from build123d import *

# Parameters (mm, degrees)
SKETCH2_R               = 5
BOSS_EXTRUDE1_DEPTH     = 5
SKETCH3_R               = 12.5
BOSS_EXTRUDE2_DEPTH     = 1.5
CUT_EXTRUDE1_DEPTH      = 22.943108257
CUT_EXTRUDE1_DEPTH_BACK = 22.943108257
SKETCH5_R               = 4.4
BOSS_EXTRUDE3_DEPTH     = 4
CUT_EXTRUDE2_DEPTH      = 25.525496937
SKETCH7_R               = 1.25
CUT_EXTRUDE3_DEPTH      = 23.210438987
SKETCH9_R               = 2
CUT_EXTRUDE4_DEPTH      = 22.089096709


with BuildPart() as part:
    # Sketch2 → Boss-Extrude1 (new, symmetric)
    with BuildSketch(Plane(origin=(0, 0, 0), x_dir=(1, 0, 0), z_dir=(0, 1, 0))):
        with Locations(Location((0, 0, 0), (0, 0, 270))):
            Circle(SKETCH2_R)
    extrude(amount=BOSS_EXTRUDE1_DEPTH, both=True)

    # Sketch3 → Boss-Extrude2 (add)
    with BuildSketch(Plane(origin=(0, 5, 0), x_dir=(1, 0, 0), z_dir=(0, 1, 0))):
        with Locations(Location((0, 0, 0), (0, 0, 270))):
            Circle(SKETCH3_R)
    boss_extrude2 = extrude(amount=BOSS_EXTRUDE2_DEPTH)

    # Mirror1: Boss-Extrude2 across plane
    add(boss_extrude2.mirror(Plane.ZX))

    # Sketch4 → Cut-Extrude1 (cut, two sides: drawn at the far end of the back side and taken through both)
    with BuildSketch(Plane(origin=(0, 6.5, 0), x_dir=(1, 0, 0), z_dir=(0, 1, 0)).offset(-CUT_EXTRUDE1_DEPTH_BACK)):
        with BuildLine():
            Line((-1.92, 2.56), (1.92, 2.56))
            ThreePointArc((1.92, 2.56), (0, -3.2), (-1.92, 2.56))
        make_face()
    extrude(amount=CUT_EXTRUDE1_DEPTH + CUT_EXTRUDE1_DEPTH_BACK, mode=Mode.SUBTRACT)

    # Sketch5 → Boss-Extrude3 (add)
    with BuildSketch(Plane(origin=(0, 6.5, 0), x_dir=(1, 0, 0), z_dir=(0, 1, 0))):
        with Locations(Location((0, 0, 0), (0, 0, 270))):
            Circle(SKETCH5_R)
    extrude(amount=BOSS_EXTRUDE3_DEPTH)

    # Sketch6 → Cut-Extrude2 (cut, through all)
    with BuildSketch(Plane(origin=(0, 10.5, 0), x_dir=(1, 0, 0), z_dir=(0, 1, 0))):
        with BuildLine():
            Line((-1.92, 2.56), (1.92, 2.56))
            ThreePointArc((1.92, 2.56), (0, -3.2), (-1.92, 2.56))
        make_face()
    extrude(amount=-CUT_EXTRUDE2_DEPTH, mode=Mode.SUBTRACT)

    # Sketch7 → Cut-Extrude3 (cut, through all)
    with BuildSketch(Plane.XY.offset(-2.56)):
        with Locations((0, 8.3)):
            Circle(SKETCH7_R)
    extrude(amount=-CUT_EXTRUDE3_DEPTH, mode=Mode.SUBTRACT)

    # Sketch9 → Cut-Extrude4 (cut, through all)
    with BuildSketch(Plane.XZ.offset(-5)):
        with Locations(Location((0, 8, 0), (0, 0, 270))):
            Circle(SKETCH9_R)
    extrude(amount=-CUT_EXTRUDE4_DEPTH, mode=Mode.SUBTRACT)


solid = part.part
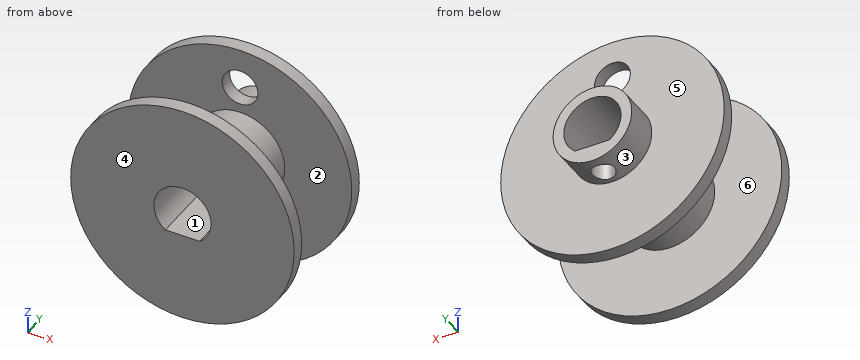
Input: part model. Units: mm. Frame: model coordinates. Face numbers are marked on the shaded views. A direction names the side the tool comes from. Round coordinates to 2 decimals unless told otherwise and drop trailing zeros. Order: outer loops, then holes, each group sorted by start corner. A loop starts at its lowest first (then second) coordinate and runs counter-clockwise, first axis right, second up. Notation, with made-up numbers: (60, 4.5) - (75, 4.5) arc R22 cw to (75, 35.5) - close; hole circle Ø9 at (80, 45). An arc over 180 degrees is marked (long way). Answer as a JSON object with one key per item and string values. Group by question number.
(1) Material intervals for probe 1 along Y at (x, z) = (2, -10.5); probe 2 along Y at (x, z) = (0, -3.85); probe 3 along Z at (x, y) = (-1.75, 6), sorted ascending. Write a range as from..to.
(2) Cut plane D-D (z = 8). Return loops of the section in (x, y), then the cut area to 3 significant figures.
(3) Cut plane B-B (z = 0). Return loops of the section in (x, y), then the cut area to 3 significant figures.
(4) Cut plane A-A (x = 7.5). Return loops of the section in (y, z).
(5) Draft query along X for the marked faces 1, 2 and 3. Return one class per face: released by +X, released by -X, zero draft, split by the parting line, or undercut.
(6) Reachability of the marked faces 4, 5 and 6 from +Z, -Z, +X, -X, +Y, -Y: full face, straight path, thin tool, end or side. Return the list, or none.
(7) Pin query (flat end, axial travel): P1, Ø3, axis at x = 0, y = 8.3, coming from the +Z side; P2, Ø1.5, axis at y = -0.5, z = -3.5, coming from the -X side; P3, Ø6.5, axis at x = 0, z = 8, coming from the +Y side; P4, Ø1.5, axis at x = -7.5, y = 3, coming from the +Z side. Return the tip coordinate at first contact, or that it passes through.
(8) Cut plane C-C (x = 0). Return loops of the section in (y, z).
Here are the results:
{
 "1": {"probe 1": "y = -6.5..-5, 5..6.5", "probe 2": "y = -6.5..7.05, 9.55..10.5", "probe 3": "z = -12.38..-2.56, 2.68..7.03, 8.97..12.38"},
 "2": {"outline": "(-9.6, -6.5) - (9.6, -6.5) - (9.6, -5) - (-9.6, -5) - close; (-9.6, 5) - (-2, 5) - (-2, 6.5) - (-9.6, 6.5) - close; (2, 5) - (9.6, 5) - (9.6, 6.5) - (2, 6.5) - close", "area": "51.6 mm^2"},
 "3": {"outline": "(-12.5, -6.5) - (-3.2, -6.5) - (-3.2, 10.5) - (-4.4, 10.5) - (-4.4, 6.5) - (-12.5, 6.5) - (-12.5, 5) - (-5, 5) - (-5, -5) - (-12.5, -5) - close; (3.2, -6.5) - (12.5, -6.5) - (12.5, -5) - (5, -5) - (5, 5) - (12.5, 5) - (12.5, 6.5) - (4.4, 6.5) - (4.4, 10.5) - (3.2, 10.5) - close", "area": "101 mm^2"},
 "4": {"outline": "(-6.5, -10) - (-5, -10) - (-5, 10) - (-6.5, 10) - close; (5, -10) - (6.5, -10) - (6.5, 10) - (5, 10) - close"},
 "5": {"face 1": "undercut", "face 2": "zero draft", "face 3": "split by the parting line"},
 "6": {"face 4": "+Z, -Z, +X, -X, -Y", "face 5": "+Y", "face 6": "none"},
 "7": {"P1": "stops at z = 4.4", "P2": "stops at x = -4.18", "P3": "stops at y = 6.5", "P4": "passes through"},
 "8": {"outline": "(-6.5, -12.5) - (-5, -12.5) - (-5, -5) - (5, -5) - (5, -12.5) - (6.5, -12.5) - (6.5, -4.4) - (7.05, -4.4) - (7.05, -2.56) - (-6.5, -2.56) - close; (-6.5, 3.2) - (10.5, 3.2) - (10.5, 4.4) - (6.5, 4.4) - (6.5, 6) - (5, 6) - (5, 5) - (-5, 5) - (-5, 12.5) - (-6.5, 12.5) - close; (5, 10) - (6.5, 10) - (6.5, 12.5) - (5, 12.5) - close; (9.55, -4.4) - (10.5, -4.4) - (10.5, -2.56) - (9.55, -2.56) - close"}
}
